Check sheet for the drawn part. Datum: minimum x, y, z corner. Units: mm. A direction names the side the tool comes from. Give positions to 0.01 mm unless a question says otherwise; leave off trailing zeros. Order: outer loops, then holes, each group sorted by start corner. A loop starts at its lowest first (then second) coordinate and runs counter-clockwise, first axis right, second up.
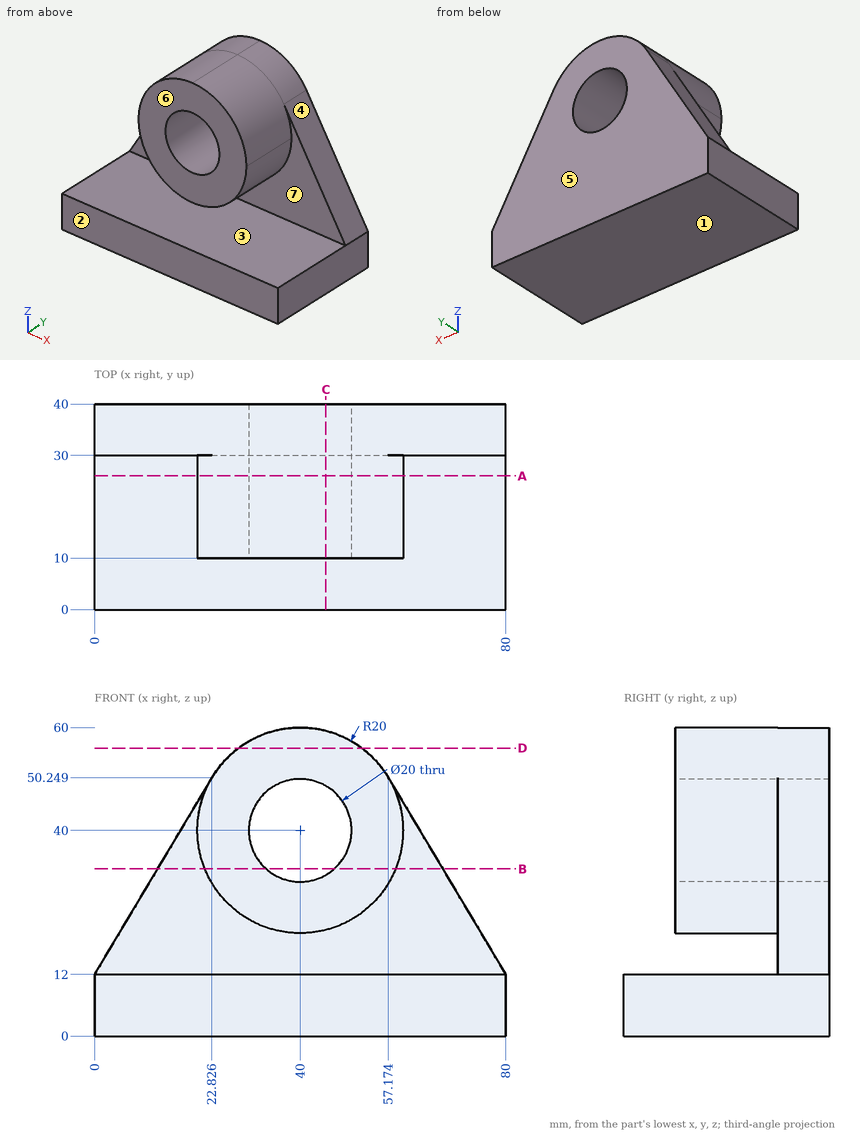
(1) Release check for a two-part mould opening along Z. For the marked faces 1, 2, 3 and 4 record: pulls with the +Z half, pulls with the -Z half, needs draft (parallel to the pull), parting line crosses it, or undercut.
Solved:
face 1: pulls with the -Z half
face 2: needs draft
face 3: undercut
face 4: pulls with the +Z half
(2) Set-up check for the marked faces 5, 6 and 7: record each of +Z, -Z, +X, -X, +Y, -Y from which the full face is reachable in a straight line by a thin tool's end or side.
Solved:
face 5: +Z, -Z, +X, -X, +Y
face 6: +Z, +X, -X, -Y
face 7: -Y
(3) Scan lines: line 1 (Z direction, x = 40, y = 24.5); line 2 (Z direction, x = 40, y = 33); line 3 (Z direction, x = 35.5, y = 28). Record each from-to range of solid material in increasing order.
Solved:
line 1: z = 0 to 12, 20 to 30, 50 to 60
line 2: z = 0 to 30, 50 to 60
line 3: z = 0 to 12, 20.51 to 31.07, 48.93 to 59.49
(4) Go/stop test with flat-tipped pins: pin 1 (8 mm diameter, centred on x = 44.5, z = 43, fed in from -Y); pin 2 (20 mm diameter, centred on x = 44, z = 38, fed in from -Y); pin 3 (9 mm diameter, centred on x = 57.5, y = 21.5, fed in from +Z); pin 4 (2 mm diameter, centred on x = 26, z = 18.5, fed in from -Y). Record where each tip stops, or that it passes through.
Solved:
pin 1: passes through
pin 2: stops at y = 10
pin 3: stops at z = 55.2
pin 4: stops at y = 30
(5) Section check C-C, the plane x = 45. Enter the section's corners in (y, z) (1 decimal).
Solved:
outline: (0, 0) - (40, 0) - (40, 31.3) - (10, 31.3) - (10, 20.6) - (30, 20.6) - (30, 12) - (0, 12) - close; (10, 48.7) - (40, 48.7) - (40, 59.4) - (10, 59.4) - close
(6) Section check B-B, the plane z = 32.5. Enter the section's corners in (x, y) (1 decimal), then the cut area to 3 significant figures.
Solved:
outline: (12.2, 30) - (21.5, 30) - (21.5, 10) - (33.4, 10) - (33.4, 40) - (12.2, 40) - close; (46.6, 10) - (58.5, 10) - (58.5, 30) - (67.8, 30) - (67.8, 40) - (46.6, 40) - close
area: 900 mm2
(7) Section check D-D, the plane z = 56. Enter the section's corners in (x, y), then the cut area to 3 significant figures.
Solved:
outline: (28, 10) - (52, 10) - (52, 40) - (28, 40) - close
area: 720 mm2
(8) Section check A-A, the plane y = 26. Enter the section's corners in (x, z), then the cut area to 3 significant figures.
Solved:
outline: (0, 0) - (80, 0) - (80, 12) - (0, 12) - close; circle Ø40 at (40, 40); hole circle Ø20 at (40, 40)
area: 1,900 mm2
